```python
from build123d import *

# Parameters (mm, degrees)
F0_W     = 38.1
F0_H     = 38.1
F1_DEPTH = 0.79375
F2_W     = 38.1
F2_H     = 38.1
F2_W_2   = 34.925
F2_H_2   = 34.925
F3_DEPTH = 5.08
F4_R     = 1.27
F5_DEPTH = 0.396875
F4_W     = 1.27
F4_H     = 29.845
F4_W_2   = 3.175
F4_H_2   = 17.203249
F6_DEPTH = 4.445


with BuildPart() as f1:
    # F0 (on Top) → F1 (new body)
    with BuildSketch(Plane.XY):
        with Locations((-1.697784, 5.910519)):
            Rectangle(F0_W, F0_H)
    extrude(amount=F1_DEPTH)

    # F2 (on face) → F3 (join)
    with BuildSketch(Plane.XY.offset(0.79375)):
        with Locations((-1.697784, 5.910519)):
            Rectangle(F2_W, F2_H)
        with Locations((-1.697784, 5.910519)):
            Rectangle(F2_W_2, F2_H_2, mode=Mode.SUBTRACT)
    extrude(amount=F3_DEPTH)

    # F4 (on face) → F5 (cut)
    with BuildSketch(Plane.XY.offset(0.79375)):
        with Locations((-16.620284, -5.438046)):
            Circle(F4_R)
        with Locations((6.874716, 17.319087)):
            Circle(F4_R)
    extrude(amount=-F5_DEPTH, mode=Mode.SUBTRACT)

    # F4 (on face) → F6 (join)
    with BuildSketch(Plane.XY.offset(0.79375)):
        with Locations((-13.445284, 3.370519)):
            Rectangle(F4_W, F4_H)
        Polygon((-2.015284, 23.373019), (-3.285284, 23.373019), (-3.285284, 18.175395), (-6.460284, 18.175395), (-7.730284, 18.175395), (-7.730284, -6.471981), (-6.460284, -6.471981), (-6.460284, -1.567854), (-3.285284, -1.567854), (-2.015284, -1.567854), (-2.015284, 16.905395), (-2.015284, 18.175395), align=None)
        with Locations((-4.872784, 8.30377)):
            Rectangle(F4_W_2, F4_H_2, mode=Mode.SUBTRACT)
        Polygon((3.064716, 8.161802), (3.064716, -11.551981), (4.334716, -11.551981), (4.334716, 6.891802), (10.071768, 6.891802), (10.071768, 8.161802), (4.334716, 8.161802), align=None)
        Polygon((3.386088, 23.373019), (3.064716, 23.373019), (3.064716, 13.241802), (4.334716, 13.241802), (10.684716, 13.241802), (10.684716, 14.511802), (10.684716, 18.293019), (9.414716, 18.293019), (9.414716, 14.511802), (4.334716, 14.511802), (4.334716, 23.373019), align=None)
    extrude(amount=F6_DEPTH)


solid = f1.part
```
Build history of the part. All positions in model axes, mm. A direction names the side the tool comes from. Round coordinates to 2 decimals unless told otherwise and drop trailing zeros. Loops run counter-clockwise (first coordinate to the right, second up) from the corner with the lowest first, then second, coordinate; pieces in that order, holes last. Notation, with made-up numbers: M 39.5,83 L 49.5,83 A10 ccw 49.5,97 Z; hole C 7,34 d9. An arc over 180 degrees is marked long. Answer as CSV lines item,"result".
1. Cut at B-B on x = -11. Write the cut outline in (y, z), then the cut area to 3 significant figures.
Resolved:
outline,"M -13.14,0 L 24.96,0 L 24.96,5.87 L 23.37,5.87 L 23.37,0.79 L -11.55,0.79 L -11.55,5.87 L -13.14,5.87 Z"
area,"46.4 mm²"
2. Cut at C-C on z = 4.55. Count the separate pieces of the cut face and the enclosed holes in it, then the cut area to 3 significant figures.
Resolved:
separate pieces,"1"
enclosed holes,"2"
area,"399 mm²"
3. Cut at D-D on y = -2.5. Write the cut outline in (x, z), then the cut area to 3 significant figures.
Resolved:
outline,"M -20.75,0 L 17.35,0 L 17.35,5.87 L 15.76,5.87 L 15.76,0.79 L 4.33,0.79 L 4.33,5.24 L 3.06,5.24 L 3.06,0.79 L -6.46,0.79 L -6.46,5.24 L -7.73,5.24 L -7.73,0.79 L -12.81,0.79 L -12.81,5.24 L -14.08,5.24 L -14.08,0.79 L -19.16,0.79 L -19.16,5.87 L -20.75,5.87 Z"
area,"63.3 mm²"
4. Two-plate mould, pull along Y, no slides. Class faces 3 (the flat face through (-2, -11.552, 3)), 4 (the flat face through (17.352, 6, 3)), 5 (the flat face through (-2, 24.961, 3)): released by +Y, released by -Y, zero draft, split by the parting line, or undercut.
Resolved:
face 3,"undercut"
face 4,"zero draft"
face 5,"released by +Y"
5. Flat gauge pins, fed straight in: P1, Ø1, axis at x = -13.5, y = 5.5, coming from the +Z side; P2, Ø0.8, axis at x = 7, y = 18, coming from the +Z side. Where does each tip first touch, or does it go through?
Resolved:
P1,"stops at z = 5.24"
P2,"stops at z = 0.4"
6. Cut at A-A on y = 7.5. Write the cut outline in (x, z).
Resolved:
outline,"M -20.75,0 L 17.35,0 L 17.35,5.87 L 15.76,5.87 L 15.76,0.79 L 10.07,0.79 L 10.07,5.24 L 3.06,5.24 L 3.06,0.79 L -2.02,0.79 L -2.02,5.24 L -3.29,5.24 L -3.29,0.79 L -6.46,0.79 L -6.46,5.24 L -7.73,5.24 L -7.73,0.79 L -12.81,0.79 L -12.81,5.24 L -14.08,5.24 L -14.08,0.79 L -19.16,0.79 L -19.16,5.87 L -20.75,5.87 Z"
7. 3-axis set-ups, long thin cutter, end or side, ignore diameter. For faces 1 (the flat face through (-2, -13.139, 3)), 2 (the flat face through (-5, 8, 0.794)): which of +Z, -Z, +X, -X, +Y, -Y reach the whole face in a straight line?
Resolved:
face 1,"+Z, -Z, +X, -X, -Y"
face 2,"+Z"
8. Wall check: probe 1 along X at (y, z) = (22, 1.35); probe 2 along X at (y, z) = (7, 1.4); probe 3 along X at (y, z) = (3.5, 1.05). Give the ranges that are in metal, low to high. Write a range as [from, to].
Resolved:
probe 1,"x = [-20.75, -19.16], [-3.29, -2.02], [3.06, 4.33], [15.76, 17.35]"
probe 2,"x = [-20.75, -19.16], [-14.08, -12.81], [-7.73, -6.46], [-3.29, -2.02], [3.06, 10.07], [15.76, 17.35]"
probe 3,"x = [-20.75, -19.16], [-14.08, -12.81], [-7.73, -6.46], [-3.29, -2.02], [3.06, 4.33], [15.76, 17.35]"
